from build123d import *

# Parameters (mm, degrees)
F1_DEPTH = 4
F2_DEPTH = 2


with BuildPart() as f1:
    # F0 (on Top) → F1 (new body)
    with BuildSketch(Plane.XY):
        Polygon((-2.15507, -42.513097), (-0.012324, -42.513097), (2.128266, -42.513097), (8.551832, -41.649458), (16.529186, -39.171592), (23.748692, -35.252986), (30.037865, -30.063322), (35.227457, -23.774077), (39.146422, -16.554931), (41.624073, -8.575349), (42.487568, -2.151782), (42.487568, -0.011192), (42.487568, 2.131554), (41.624073, 8.553324), (39.146422, 16.530678), (35.227457, 23.749824), (30.037865, 30.039356), (23.748692, 35.228948), (16.529186, 39.147554), (8.551832, 41.625565), (2.128266, 42.486903), (-0.012324, 42.486903), (-2.15507, 42.486903), (-8.578637, 41.625565), (-16.556206, 39.147554), (-23.775352, 35.228948), (-30.064598, 30.039356), (-35.254262, 23.749824), (-39.172867, 16.530678), (-41.650734, 8.553324), (-42.512432, 2.131554), (-42.512432, -0.011192), (-42.512432, -2.151782), (-41.650734, -8.575349), (-39.172867, -16.554931), (-35.254262, -23.774077), (-30.064598, -30.063322), (-23.775352, -35.252986), (-16.556206, -39.171592), (-8.578637, -41.649458), align=None)
        Polygon((-32.156461, 7.865187), (-31.973198, 8.547215), (-14.778227, -29.622735), (-15.790021, -29.11779), (-18.683142, -27.324179), (-22.221601, -24.528584), (-25.344771, -21.286472), (-28.007842, -17.644702), (-30.162087, -13.646215), (-31.758743, -9.343618), (-32.751061, -4.78359), (-33.092255, -1.204202), (-33.092255, -0.011192), (-33.092255, 1.957992), align=None, mode=Mode.SUBTRACT)
        Polygon((-8.438135, -32.020684), (-9.163643, -31.812051), (-0.012324, -11.515471), (9.128933, -31.813992), (8.401628, -32.022625), (2.272361, -33.09292), (-0.012324, -33.09292), (-2.119855, -33.09292), align=None, mode=Mode.SUBTRACT)
        Polygon((15.763073, -29.11779), (14.753686, -29.622735), (31.967882, 8.475347), (32.147192, 7.798709), (33.065307, 2.112149), (33.065307, -0.011192), (33.065307, -1.204202), (32.722496, -4.78359), (31.730358, -9.343618), (30.13345, -13.646215), (27.979205, -17.644702), (25.31829, -21.286472), (22.194904, -24.528584), (18.656481, -27.324179), align=None, mode=Mode.SUBTRACT)
        Polygon((-0.012324, 11.140574), (-9.317441, 31.741192), (-8.580434, 31.957874), (-2.15507, 33.064642), (-0.012324, 33.064642), (2.311529, 33.064642), (8.543927, 31.959311), (9.28309, 31.743348), align=None, mode=Mode.SUBTRACT)
        Polygon((5.602367, 0.876019), (17.744116, 27.900922), (18.615516, 27.344664), (22.618207, 24.112757), (26.095902, 20.326748), (26.706062, 19.494157), (11.45099, -14.266185), (5.565355, -1.175095), (-5.590004, -1.175095), (-11.475638, -14.266185), (-26.707461, 19.523263), (-26.101182, 20.354058), (-22.630997, 24.126053), (-18.640272, 27.34682), (-17.770777, 27.900922), (-5.590004, 0.876019), align=None, mode=Mode.SUBTRACT)
    extrude(amount=F1_DEPTH)

    # F0 (on Top) → F2 (join)
    with BuildSketch(Plane.XY):
        Polygon((18.615516, 27.344664), (17.744116, 27.900922), (5.602367, 0.876019), (-5.590004, 0.876019), (-17.770777, 27.900922), (-18.640272, 27.34682), (-22.630997, 24.126053), (-26.101182, 20.354058), (-26.707461, 19.523263), (-11.475638, -14.266185), (-5.590004, -1.175095), (5.565355, -1.175095), (11.45099, -14.266185), (26.706062, 19.494157), (26.095902, 20.326748), (22.618207, 24.112757), align=None)
        Polygon((-14.778227, -29.622735), (-31.973198, 8.547215), (-32.156461, 7.865187), (-33.092255, 1.957992), (-33.092255, -0.011192), (-33.092255, -1.204202), (-32.751061, -4.78359), (-31.758743, -9.343618), (-30.162087, -13.646215), (-28.007842, -17.644702), (-25.344771, -21.286472), (-22.221601, -24.528584), (-18.683142, -27.324179), (-15.790021, -29.11779), align=None)
        Polygon((-0.012324, -11.515471), (-9.163643, -31.812051), (-8.438135, -32.020684), (-2.119855, -33.09292), (-0.012324, -33.09292), (2.272361, -33.09292), (8.401628, -32.022625), (9.128933, -31.813992), align=None)
        Polygon((31.967882, 8.475347), (14.753686, -29.622735), (15.763073, -29.11779), (18.656481, -27.324179), (22.194904, -24.528584), (25.31829, -21.286472), (27.979205, -17.644702), (30.13345, -13.646215), (31.730358, -9.343618), (32.722496, -4.78359), (33.065307, -1.204202), (33.065307, -0.011192), (33.065307, 2.112149), (32.147192, 7.798709), align=None)
        Polygon((-8.580434, 31.957874), (-9.317441, 31.741192), (-0.012324, 11.140574), (9.28309, 31.743348), (8.543927, 31.959311), (2.311529, 33.064642), (-0.012324, 33.064642), (-2.15507, 33.064642), align=None)
    extrude(amount=F2_DEPTH)


solid = f1.part
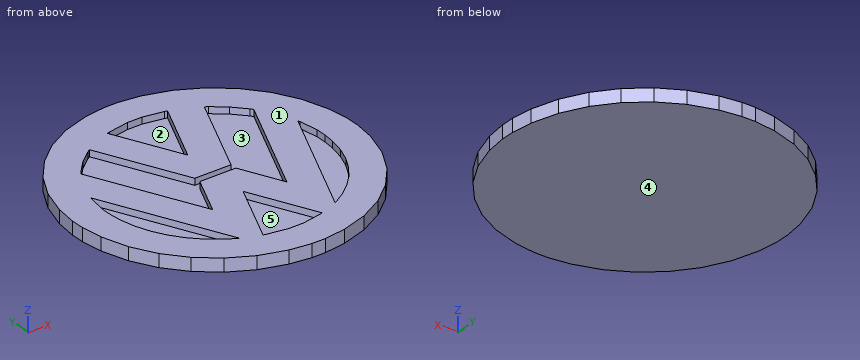
Can you work these out from the model? Positions are in its coordinate system, mm. Face numbers are marked on the shaded views. A direction names the side the tool comes from. Coordinates: 2 decimals unless noted, no trailing zeros. Write each loop counter-clockwise with the first axis right and the second up, starting at its lowest first coordinate (ties: lowest second). Pieces come first, ordered by that corner, then holes. Notation, with made-up numbers: M 51.25,-31 L 107.25,-31 A26 cw 107.25,-15 Z; hole C 55,84 d9. An arc over 180 degrees is marked long. Use one line per item in the form item = value.
Q1. If we section it at A-A (y = -25.5): Write out the boundary of the cut face in (x, z), then the cut area to 3 significant figures.
Model answer:
outline = M -33.83,0 L 33.8,0 L 33.8,4 L 20.97,4 L 20.97,2 L 16.62,2 L 16.62,4 L 6.29,4 L 6.29,2 L -6.32,2 L -6.32,4 L -16.64,4 L -16.64,2 L -20.99,2 L -20.99,4 L -33.83,4 Z
area = 228 mm^2
Q2. I need wall thicknesses on line 1 along Y through (x, z) = (-7.5, 2.1); line 2 along Y through (x, z) = (2, 3.45); line 3 along X through (y, z) = (14, 2.2). Which ranges of each line are inside material? Lowest first, please. Write a range as from..to.
Model answer:
line_1 = -41.79..-32.18, -28.12..-5.42, 5.11..27.72, 32.14..41.77
line_2 = -42.51..-33.09, -15.98..-1.18, 0.88..15.6, 33.06..42.49
line_3 = -39.96..-24.22, -11.51..-1.3, 1.28..11.5, 24.22..39.93
Q3. If we section it at C-C (z = 2.65): State how many separate pieces and enclosed holes the cut face has, then the cut area to 3 significant figures.
Model answer:
separate_pieces = 1
enclosed_holes = 5
area = 4,000 mm^2
Q4. If we section it at D-D (x = -13): Write out the boundary of the cut face in (y, z).
Model answer:
outline = M -40.28,0 L 40.25,0 L 40.25,4 L 17.32,4 L 17.32,2 L -10.88,2 L -10.88,4 L -40.28,4 Z
Q5. For the marked faces 1 and 2, which set-ups out of +Z, -Z, +X, -X, +Y, -Y let a thin tool reach every point of the face, with its end or its side?
Model answer:
face_1 = +Z, +X, -X, +Y, -Y
face_2 = +Z
Q6. For P1, Ø15, axis at x = 2, y = 19.5, coming from the +Z side; P2, Ø2, axis at x = -8, z = 2.5, coming from the -Y side; P3, Ø0.6, axis at x = 2.5, z = 3.5, coming from the +Y side, each with a flat end and sliding along its axis, tell me the tip position at first contact or that it passes through.
Model answer:
P1 = 4
P2 = -41.86
P3 = 42.48
Q7. We'd pull the mould along Y, two halves only. Please class the marked faces 3, 4 and 5: +Y half, -Y half, draft (parallel to the pull), parting line (faces both ways), or undercut.
Model answer:
face_3 = undercut
face_4 = draft
face_5 = undercut
Q8. If we section it at B-B (x = -1): Write out the boundary of the cut face in (y, z), then the cut area to 3 significant figures.
Model answer:
outline = M -42.51,0 L 42.49,0 L 42.49,4 L 33.06,4 L 33.06,2 L 13.33,2 L 13.33,4 L 0.88,4 L 0.88,2 L -1.18,2 L -1.18,4 L -13.71,4 L -13.71,2 L -33.09,2 L -33.09,4 L -42.51,4 Z
area = 258 mm^2
